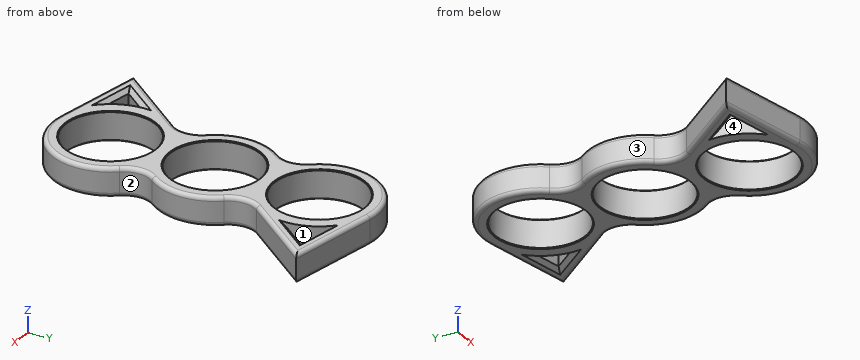
```python
from build123d import *

# Parameters (mm, degrees)
F0_R     = 10.9855
F1_DEPTH = 7
F2_SIZE  = 0.2
F3_SIZE  = 1
F4_R     = 1


with BuildPart() as f1:
    # F0 (on Top) → F1 (new body)
    with BuildSketch(Plane.XY):
        with BuildLine():
            ThreePointArc((-11.119352, 16.631889), (-9.755608, 12.7), (-11.119352, 8.768111))
            ThreePointArc((-11.119352, 8.768111), (-14.1605, 0), (-11.119352, -8.768111))
            ThreePointArc((-11.119352, -8.768111), (-9.755608, -12.7), (-11.119352, -16.631889))
            Line((-11.119352, -16.631889), (-25.4, -34.742009))
            Line((-25.4, -34.742009), (-2.788271, -39.283274))
            ThreePointArc((-2.788271, -39.283274), (12.067437, -32.809232), (11.119352, -16.631889))
            ThreePointArc((11.119352, -16.631889), (9.755608, -12.7), (11.119352, -8.768111))
            ThreePointArc((11.119352, -8.768111), (14.1605, 0), (11.119352, 8.768111))
            ThreePointArc((11.119352, 8.768111), (9.755608, 12.7), (11.119352, 16.631889))
            Line((11.119352, 16.631889), (25.4, 34.742009))
            Line((25.4, 34.742009), (2.788271, 39.283274))
            ThreePointArc((2.788271, 39.283274), (-12.067437, 32.809232), (-11.119352, 16.631889))
        make_face()
        with BuildLine():
            Line((-19.704933, -32.647388), (-14.158881, -25.614117))
            ThreePointArc((-14.158881, -25.614117), (-13.290102, -30.288041), (-10.923412, -34.41104))
            Line((-10.923412, -34.41104), (-19.704933, -32.647388))
        make_face(mode=Mode.SUBTRACT)
        with Locations((0, -25.4)):
            Circle(F0_R, mode=Mode.SUBTRACT)
        Circle(F0_R, mode=Mode.SUBTRACT)
        with Locations((0, 25.4)):
            Circle(F0_R, mode=Mode.SUBTRACT)
        with BuildLine():
            Line((19.704933, 32.647388), (14.158881, 25.614117))
            ThreePointArc((14.158881, 25.614117), (13.290102, 30.288041), (10.923412, 34.41104))
            Line((10.923412, 34.41104), (19.704933, 32.647388))
        make_face(mode=Mode.SUBTRACT)
    extrude(amount=F1_DEPTH)

    # F2
    f2_edges = [f1.edges().sort_by_distance(p)[0] for p in [
        (-10.9855, 25.4, 7),
        (-10.9855, 0, 7),
        (-10.9855, -25.4, 7),
        (-10.9855, 25.4, 0),
        (-10.9855, 0, 0),
        (-10.9855, -25.4, 0),
    ]]
    chamfer(f2_edges, length=F2_SIZE)

    # F3
    f3_edges = [f1.edges().sort_by_distance(p)[0] for p in [
        (15.314172, 33.529214, 7),
        (16.931907, 29.130753, 7),
        (15.314172, 33.529214, 0),
        (16.931907, 29.130753, 0),
        (-16.931907, -29.130753, 7),
        (-15.314172, -33.529214, 7),
        (-16.931907, -29.130753, 0),
        (-15.314172, -33.529214, 0),
    ]]
    chamfer(f3_edges, length=F3_SIZE)

    # F4
    f4_edges = [f1.edges().sort_by_distance(p)[0] for p in [
        (-14.1605, 0, 0),
        (12.067437, -32.809232, 0),
        (-12.067437, 32.809232, 7),
        (18.259676, 25.686949, 7),
    ]]
    fillet(f4_edges, radius=F4_R)


solid = f1.part
```
The model under review builds one solid part; all positions refer to its coordinate system, in mm. Face numbers are marked on the shaded views. Give positions to 0.01 mm unless a question says otherwise; leave off trailing zeros. Loops run counter-clockwise (first coordinate to the right, second up) from the corner with the lowest first, then second, coordinate; pieces in that order, holes last. Notation, with made-up numbers: (38, 15) -> (53, 15) arc R14 cw to (53, 28) -> close; hole circle Ø6 at (-25.5, 34.25). An arc over 180 degrees is marked (long way). Use CSV: the item, a comma, the result in double quotes.
1. Consider section C-C, the plane y = 0. Write out the cut boundary in (x, z), then the cut area to 3 significant figures.
Result:
outline,"(-14.16, 1) arc R1 ccw to (-13.16, 0) -> (-11.19, 0) -> (-10.99, 0.2) -> (-10.99, 6.8) -> (-11.19, 7) -> (-13.16, 7) arc R1 ccw to (-14.16, 6) -> close; (10.99, 0.2) -> (11.19, 0) -> (13.16, 0) arc R1 ccw to (14.16, 1) -> (14.16, 6) arc R1 ccw to (13.16, 7) -> (11.19, 7) -> (10.99, 6.8) -> close"
area,"43.5 mm²"
2. To check wall thickness, follow probe 1 along Y at (x, z) = (0, 2.5); probe 2 along Y at (x, z) = (-9, 3.75); probe 3 along X at (y, z) = (-32, 2.25). State the ranges of each line that lie inside material, in increasing order. Write a range as from..to.
Result:
probe 1,"y = -39.56..-36.39, -14.41..-10.99, 10.99..14.41, 36.39..39.56"
probe 2,"y = -38.04..-31.7, -19.1..-6.3, 6.3..19.1, 31.7..36.33"
probe 3,"x = -23.24..-19.19, -12.53..-8.78, 8.78..12.53"
3. For P1, Ø4, axis at x = -6.5, z = 3.5, coming from the +Y side; P2, Ø1, axis at y = 25.5, z = 3.5, coming from the -X side; P3, Ø3, axis at y = -12, z = 1, coming from the -X side, all flat-tipped, find the tip position at first contact; note any pin that passes through.
Result:
P1,"stops at y = 38.83"
P2,"stops at x = -14.16"
P3,"stops at x = -10.15"
4. The part is to be moulded in two halves that separate along X. For the marked faces 1, 2, 3 and 4, say which applies: +X half, -X half, draft (parallel to the pull), parting line (faces both ways), or undercut.
Result:
face 1,"undercut"
face 2,"+X half"
face 3,"-X half"
face 4,"undercut"
5. Consider section A-A, the plane z = 2.5. Write out the cut boundary in (x, y).
Result:
outline,"(-25.4, -34.74) -> (-2.79, -39.28) arc R14.16 ccw to (11.12, -16.63) arc R6.35 cw to (11.12, -8.77) arc R14.16 ccw to (11.12, 8.77) arc R6.35 cw to (11.12, 16.63) -> (25.4, 34.74) -> (2.79, 39.28) arc R14.16 ccw to (-11.12, 16.63) arc R6.35 cw to (-11.12, 8.77) arc R14.16 ccw to (-11.12, -8.77) arc R6.35 cw to (-11.12, -16.63) -> close; hole (-19.7, -32.65) -> (-10.92, -34.41) arc R14.16 cw to (-14.16, -25.61) -> close; hole circle Ø21.97 at (0, -25.4); hole circle Ø21.97 at (0, 0); hole circle Ø21.97 at (0, 25.4); hole (10.92, 34.41) arc R14.16 cw to (14.16, 25.61) -> (19.7, 32.65) -> close"
6. Consider section B-B, the plane x = 0. Count the separate pieces of the cut face and the enclosed holes in it, then the cut area to 3 significant figures.
Result:
separate pieces,"4"
enclosed holes,"0"
area,"91.4 mm²"
